Can you work these out from the model? Positions are in its coordinate system, mm. A direction names the side the tool comes from. Coordinates: 2 decimals unless noted, no trailing zeros. Order: outer loops, then holes, each group sorted by start corner. A loop starts at its lowest first (then second) coordinate and runs counter-clockwise, first axis right, second up.
```python
from build123d import *

# Parameters (mm, degrees)
F0_R     = 13.46689
F1_DEPTH = 7
F2_R     = 0.6
F3_R     = 15.865442
F4_DEPTH = 4
F5_R     = 0.5


with BuildPart() as f1:
    # F0 (on Top) → F1 (new body)
    with BuildSketch(Plane.XY):
        Circle(F0_R)
    extrude(amount=F1_DEPTH)

    # F2
    f2_edges = [f1.edges().sort_by_distance(p)[0] for p in [
        (-13.46689, 0, 7),
    ]]
    fillet(f2_edges, radius=F2_R)

    # F3 (on Top) → F4 (join)
    with BuildSketch(Plane.XY):
        Circle(F3_R)
    extrude(amount=F4_DEPTH)

    # F5
    f5_edges = [f1.edges().sort_by_distance(p)[0] for p in [
        (-15.865442, 0, 4),
    ]]
    fillet(f5_edges, radius=F5_R)


solid = f1.part
```
1. Imagine slicing it at C-C on z = 1. Please give me the cut outline in (x, y).
Completed:
outline: circle Ø31.73 at (0, 0)
2. Imagine slicing it at D-D on z = 4.75. Please give me the cut outline in (x, y).
Completed:
outline: circle Ø26.93 at (0, 0)
3. I'm going to push flat-ended pins straight in: pin 1 (12 mm diameter, centred on x = -6.5, y = 0.5, fed in from -Z); pin 2 (1 mm diameter, centred on y = -3, z = 2, fed in from +X); pin 3 (1 mm diameter, centred on y = -4, z = 5.5, fed in from -X). Where does each tip first touch, or does it pass through?
Completed:
pin 1: stops at z = 0
pin 2: stops at x = 15.67
pin 3: stops at x = -13
4. Please list where these lines run through material, in increasing order: probe 1 along Y at (x, z) = (0.5, 2); probe 2 along Y at (x, z) = (13, 1); probe 3 along Z at (x, y) = (-8.5, 11).
Completed:
probe 1: y = -15.86 to 15.86
probe 2: y = -9.09 to 9.09
probe 3: z = 0 to 4
5. Imagine slicing it at A-A on x = 0. Please give me the cut outline in (y, z).
Completed:
outline: (-15.87, 0) - (15.87, 0) - (15.87, 3.5) arc R0.5 ccw to (15.37, 4) - (13.47, 4) - (13.47, 6.4) arc R0.6 ccw to (12.87, 7) - (-12.87, 7) arc R0.6 ccw to (-13.47, 6.4) - (-13.47, 4) - (-15.37, 4) arc R0.5 ccw to (-15.87, 3.5) - close
6. On a 3-axis mill with a long thin cutter (end or side, diameter ignored), from which of +Z, -Z, +X, -X, +Y, -Y can I reach the whole of each face in a straight line? I mean faces 1 (the cylindrical face through (-3.44, -15.49, 1.73)), 2 (the flat face through (0, -14, 4)). Say none if no direction works.
Completed:
face 1: +Z, -Z
face 2: +Z
